from build123d import *

# Parameters (mm, degrees)
RESSALTO_EXTRUS_O1_DEPTH = 0.55
ESBO_O2_R                = 2.69
ESBO_O2_R_2              = 1.4
RESSALTO_EXTRUS_O2_DEPTH = 11.45


with BuildPart() as part:
    # Esboço1 → Ressalto-extrusão1 (new body)
    with BuildSketch(Plane(origin=(0, 0, 0), x_dir=(1, 0, 0), z_dir=(0, 1, 0))):
        Polygon((2.480405511, -2.738781085), (3.612056751, 0.778703642), (1.13165124, 3.517484727), (-2.480405511, 2.738781085), (-3.612056751, -0.778703642), (-1.13165124, -3.517484727), align=None)
    extrude(amount=RESSALTO_EXTRUS_O1_DEPTH)

    # Esboço2 → Ressalto-extrusão2 (add)
    with BuildSketch(Plane(origin=(0, 0.55, 0), x_dir=(1, 0, 0), z_dir=(0, 1, 0))):
        with Locations(Location((0, 0, 0), (0, 0, 270))):
            Circle(ESBO_O2_R)
        with Locations(Location((0, 0, 0), (0, 0, 270))):
            Circle(ESBO_O2_R_2, mode=Mode.SUBTRACT)
    extrude(amount=RESSALTO_EXTRUS_O2_DEPTH)


solid = part.part
Geometry check sheet. Reference: the model listing, model coordinates, mm. A direction names the side the tool comes from. Coordinates: 2 decimals unless noted, no trailing zeros. Order: outer loops, then holes, each group sorted by start corner. A loop starts at its lowest first (then second) coordinate and runs counter-clockwise, first axis right, second up. Notation, with made-up numbers: (-36.5, 33) - (-5.5, 33) arc R16 cw to (-5.5, 63) - close; hole circle Ø11 at (68, 71.5). An arc over 180 degrees is marked (long way). One line per item, written item: value.
(1) Release check for a two-part mould opening along Z. For faces 3 (the face through (-3, 0.55, 0)), 4 (the face through (0, 0.55, 0)), 5 (the face through (2.39, 0.27, -2.13)) record: +Z half, -Z half, draft (parallel to the pull), parting line (faces both ways), or undercut.
Data:
face 3: draft
face 4: undercut
face 5: -Z half
(2) Access from +Z, -Z, +X, -X, +Y, -Y to the whole of each face (thin tool, end or side, straight path). Record for faces 1 (the face through (2.268, 6.195, 1.446)), 2 (the face through (-2.39, 0.27, 2.13)).
Data:
face 1: +Y
face 2: +Z, -X, +Y, -Y
(3) Sectioned sample at C-C (x = 0). Enter the section's corners in (y, z), and give its area (3 significant figures).
Data:
outline: (0, -3.27) - (0.55, -3.27) - (0.55, -2.69) - (12, -2.69) - (12, -1.4) - (0.55, -1.4) - (0.55, 1.4) - (12, 1.4) - (12, 2.69) - (0.55, 2.69) - (0.55, 3.27) - (0, 3.27) - close
area: 33.1 mm^2
(4) Sectioned sample at A-A (z = 2). Enter the section's corners in (x, y), and give its area (3 significant figures).
Data:
outline: (-2.51, 0) - (2.72, 0) - (2.72, 0.55) - (1.8, 0.55) - (1.8, 12) - (-1.8, 12) - (-1.8, 0.55) - (-2.51, 0.55) - close
area: 44.1 mm^2
(5) Depth check by flat-ended pin: pin 1 Ø2 at (y, z) = (8.5, 0) entering from -X; pin 2 Ø1.4 at (x, z) = (-0.5, 0) entering from +Y; pin 3 Ø4 at (x, y) = (-2, 1.5) entering from -Z. Enter the tip coordinate at first touch or a pass-through.
Data:
pin 1: stops at x = -2.69
pin 2: stops at y = 0.55
pin 3: stops at z = -3.22
(6) Thickness scan on probe 1 along X at (y, z) = (6.75, 0); probe 2 along Y at (x, z) = (3, 1); probe 3 along Z at (x, y) = (-0.75, 9.75). Record the ranges inside material, lowest first. Write a range as from..to.
Data:
probe 1: x = -2.69..-1.4, 1.4..2.69
probe 2: y = 0..0.55
probe 3: z = -2.58..-1.18, 1.18..2.58
(7) Sectioned sample at B-B (y = 5). Enter the section's corners in (x, z).
Data:
outline: circle Ø5.38 at (0, 0); hole circle Ø2.8 at (0, 0)
(8) Sectioned sample at D-D (z = -1.75). Enter the section's corners in (x, y).
Data:
outline: (-2.8, 0) - (2.73, 0) - (2.73, 0.55) - (2.04, 0.55) - (2.04, 12) - (-2.04, 12) - (-2.04, 0.55) - (-2.8, 0.55) - close
